Input: part model. Units: mm. Frame: model coordinates. A direction names the side the tool comes from. Round coordinates to 2 decimals unless told otherwise and drop trailing zeros. Write each loop counter-clockwise with the first axis right and the second up, starting at its lowest first coordinate (ties: lowest second). Pieces come first, ordered by that corner, then holes. Notation, with made-up numbers: M -33,66 L -11,66 A11 ccw -11,83 Z; hole C 44,45.25 d5. An arc over 180 degrees is marked long. Use one line per item in the form item = value. Start each with the question number.
```python
from build123d import *

# Parameters (mm, degrees)
EXTRUIR_L_MINA1_DEPTH             = 10
REDONDEO3_R                       = 2
EXTRUIR_L_MINA2_DEPTH             = 5
REDONDEO4_R                       = 3
CROQUIS2_R                        = 1.5
CORTAR_EXTRUIR1_DEPTH             = 10
CROQUIS5_W                        = 13.2
CROQUIS5_H                        = 24.3
CROQUIS5_W_2                      = 9.2
CROQUIS5_H_2                      = 20.3
EXTRUIR_L_MINA3_DEPTH             = 3.5
EXTRUIR_L_MINA3_DIRECTION_2_REACH = 51.752
CROQUIS7_W                        = 10
CROQUIS7_H                        = 2
SALIENTE_EXTRUIR1_DEPTH           = 6
CORTAR_EXTRUIR2_DEPTH             = 50.751884386
CORTAR_EXTRUIR2_DEPTH_BACK        = 50.751884386
CROQUIS8_R                        = 1.5
EXTRUIR_L_MINA4_DEPTH             = 2
REDONDEO5_R                       = 3


with BuildPart() as part:
    # Croquis1 → Extruir-Lámina1 (new body)
    with BuildSketch(Plane.XY):
        Polygon((-2.15, 0), (0, 0), (7.5, 0), (7.5, 12), (32.5, 12), (32.5, 0), (40, 0), (41, 0), (41, 2), (40, 2), (34.5, 2), (34.5, 14), (5.5, 14), (5.5, 2), (0, 2), (-2.15, 2), align=None)
    extrude(amount=-EXTRUIR_L_MINA1_DEPTH)

    # Redondeo3
    redondeo3_edges = [part.edges().sort_by_distance(p)[0] for p in [
        (5.5, 14, -5),
        (34.5, 14, -5),
    ]]
    fillet(redondeo3_edges, radius=REDONDEO3_R)

    # Croquis3 → Extruir-Lámina2 (add, symmetric)
    with BuildSketch(Plane(origin=(20, 0, 0), x_dir=(0, 0, -1), z_dir=(1, 0, 0))):
        Polygon((23.5, 0), (23.5, 12), (-13.5, 12), (-13.5, 0), (-15.5, 0), (-15.5, 14), (25.5, 14), (25.5, 0), align=None)
    extrude(amount=EXTRUIR_L_MINA2_DEPTH, both=True)

    # Redondeo4
    redondeo4_edges = [part.edges().sort_by_distance(p)[0] for p in [
        (20, 14, -25.5),
        (20, 14, 15.5),
    ]]
    fillet(redondeo4_edges, radius=REDONDEO4_R)

    # Croquis2 → Cortar-Extruir1 (cut)
    with BuildSketch(Plane(origin=(0, 2, 0), x_dir=(1, 0, 0), z_dir=(0, 1, 0))):
        with Locations(Location((2.5, 5, 0), (0, 0, 270))):
            Circle(CROQUIS2_R)
        with Locations(Location((37.5, 5, 0), (0, 0, 270))):
            Circle(CROQUIS2_R)
    extrude(amount=-CORTAR_EXTRUIR1_DEPTH, mode=Mode.SUBTRACT)

    # Croquis5 → Extruir-Lámina3 (add)
    with BuildSketch(Plane(origin=(0, 2, 0), x_dir=(1, 0, 0), z_dir=(0, 1, 0))):
        with Locations((-6.75, 1.3)):
            Rectangle(CROQUIS5_W, CROQUIS5_H)
        with Locations((-6.75, 1.3)):
            Rectangle(CROQUIS5_W_2, CROQUIS5_H_2, mode=Mode.SUBTRACT)
    extrude(amount=EXTRUIR_L_MINA3_DEPTH)

    # Extruir-Lámina3 direction 2: up to this face of the body (flat: up to its plane)
    extruir_l_mina3_direction_2_end = Plane(part.part.faces().sort_by_distance((-2.011031478, 0, -5))[0])
    # Croquis5 → Extruir-Lámina3 direction 2 (add, up to the picked face)
    with BuildSketch(Plane(origin=(0, 2, 0), x_dir=(1, 0, 0), z_dir=(0, 1, 0)), mode=Mode.PRIVATE) as extruir_l_mina3_direction_2_sk1:
        with Locations((-6.75, 1.3)):
            Rectangle(CROQUIS5_W, CROQUIS5_H)
        with Locations((-6.75, 1.3)):
            Rectangle(CROQUIS5_W_2, CROQUIS5_H_2, mode=Mode.SUBTRACT)
    extruir_l_mina3_direction_2_tool1 = split(extrude(extruir_l_mina3_direction_2_sk1.sketch, amount=-EXTRUIR_L_MINA3_DIRECTION_2_REACH, mode=Mode.PRIVATE), bisect_by=extruir_l_mina3_direction_2_end, keep=Keep.BOTH, mode=Mode.PRIVATE)
    add(extruir_l_mina3_direction_2_tool1.solids().sort_by(Axis((-6.75, 2, 10.573462), (0, -1, 0)))[0])

    # Croquis7 → Saliente-Extruir1 (add)
    with BuildSketch(Plane.ZY.offset(13.35)):
        with Locations((-5, 1)):
            Rectangle(CROQUIS7_W, CROQUIS7_H)
    extrude(amount=SALIENTE_EXTRUIR1_DEPTH)

    # Croquis8 → Cortar-Extruir2 (cut, two sides: drawn at the far end of the back side and taken through both)
    with BuildSketch(Plane(origin=(0, 2, 0), x_dir=(1, 0, 0), z_dir=(0, 1, 0)).offset(-CORTAR_EXTRUIR2_DEPTH_BACK)):
        with Locations(Location((-16, 5, 0), (0, 0, 180))):
            Circle(CROQUIS8_R)
    extrude(amount=CORTAR_EXTRUIR2_DEPTH + CORTAR_EXTRUIR2_DEPTH_BACK, mode=Mode.SUBTRACT)

    # Croquis9 → Extruir-Lámina4 (add, symmetric)
    with BuildSketch(Plane.ZY.offset(6.8)):
        Polygon((8.85, 5.5), (8.85, 6.8), (-11.45, 6.8), (-11.45, 5.5), (-13.45, 5.5), (-13.45, 8.8), (10.85, 8.8), (10.85, 5.5), align=None)
    extrude(amount=EXTRUIR_L_MINA4_DEPTH, both=True)

    # Redondeo5
    redondeo5_edges = [part.edges().sort_by_distance(p)[0] for p in [
        (-19.35, 1, -10),
        (-19.35, 1, 0),
        (41, 1, 0),
        (41, 1, -10),
    ]]
    fillet(redondeo5_edges, radius=REDONDEO5_R)


solid = part.part
```
Item 1: Cut plane C-C (x = 16.5). Output: boundary loops of the cut face in (y, z), plus the area to 3 significant figures.
Item 2: First-contact query: pin 1 (1.6 mm diameter, centred on x = -14, y = 1.5, fed in from +Z); pin 2 (6 mm diameter, centred on x = 7.5, y = 6, fed in from +Z); pin 3 (2.5 mm diameter, centred on y = 6.5, z = -5.5, fed in from -X). Flat tips, straight axial feed; report the tip coordinate or a pass-through.
Item 3: Cut plane D-D (z = -5). Give the number of separate pieces and of enclosed holes in the cut face, plus the area to 3 significant figures.
Item 4: Cut plane B-B (x = 2.5). Output: boundary loops of the cut face in (y, z).
Item 5: Draft query along X for faces 6 (the face through (-18.45, 1.01, -9.14)), 7 (the face through (41, 1, -5)), 8 (the face through (-7, 3, -11.45)), 9 (the face through (-18, 2, -5)). Return one class per face: +X half, -X half, draft (parallel to the pull), parting line (faces both ways), or undercut.
Item 6: Reachability of faces 1 (the face through (15, 10, -24)), 2 (the face through (39, 2, -4)), 3 (the face through (7, 8, 0)), 4 (the face through (15, 12.2, 10)), 5 (the face through (5.5, 7, -5)) from +Z, -Z, +X, -X, +Y, -Y: full face, straight path, thin tool, end or side. Return the list, or none.
Item 7: Cut plane A-A (z = 8). Output: boundary loops of the cut face in (x, y).
Item 8: Ray query, line 1 (X direction, y = 0.8, z = -5); line 2 (Z direction, x = -16, y = 0.85); line 3 (X direction, y = 11.5, z = -8.5). Return the intervals inside material, ascending. Write a range as from..to.
Final values:
q1.outline = M 0,-25.5 L 11,-25.5 A3 ccw 14,-22.5 L 14,12.5 A3 ccw 11,15.5 L 0,15.5 L 0,13.5 L 12,13.5 L 12,-23.5 L 0,-23.5 Z
q1.area = 126 mm^2
q2.pin_1 = 10.85
q2.pin_2 = 0
q2.pin_3 = -13.35
q3.separate_pieces = 6
q3.enclosed_holes = 0
q3.area = 153 mm^2
q4.outline = M 0,-10 L 2,-10 L 2,-6.5 L 0,-6.5 Z; M 0,-3.5 L 2,-3.5 L 2,0 L 0,0 Z
q5.face_6 = -X half
q5.face_7 = +X half
q5.face_8 = undercut
q5.face_9 = draft
q6.face_1 = -Z, -X, +Y, -Y
q6.face_2 = +Z, -Z, +X, +Y
q6.face_3 = +Z, +Y, -Y
q6.face_4 = +Z, -X, +Y, -Y
q6.face_5 = +Z, -Z, +Y
q7.outline = M -13.35,0 L -11.35,0 L -11.35,5.5 L -13.35,5.5 Z; M -8.8,6.8 L -4.8,6.8 L -4.8,8.8 L -8.8,8.8 Z; M -2.15,0 L -0.15,0 L -0.15,5.5 L -2.15,5.5 Z; M 15,12 L 25,12 L 25,14 L 15,14 Z
q8.line_1 = -19.35..-17.5, -14.5..-11.35, -2.15..1, 4..7.5, 32.5..36, 39..41
q8.line_2 = -10..-6.5, -3.5..0
q8.line_3 = 5.5..7.5, 32.5..34.5
